Verification items for the finished model (mm, model axes). Face numbers are marked on the shaded views. Coordinates: 2 decimals unless noted, no trailing zeros. Order: outer loops, then holes, each group sorted by start corner. A loop starts at its lowest first (then second) coordinate and runs counter-clockwise, first axis right, second up.
Q1. Depth check by flat-ended pin: P1, Ø6, axis at y = -25.5, z = 115.5, coming from the -X side; P2, Ø12, axis at x = 0, y = 10.5, coming from the +Z side; P3, Ø6, axis at y = -17.5, z = 46, coming from the -X side. Enter the tip coordinate at first touch or a pass-through.
Q2. Thickness scan on line 1 (Y direction, x = 0, z = 47); line 2 (X direction, y = 2.5, z = 117.5); line 3 (X direction, y = 16, z = 34.5). Record the ranges inside material, lowest first.
Q3. Draft check along Y on the marked faces 1, 2 and 3. Enter one of: pulls with the +Y half, pulls with the -Y half, needs draft (parallel to the pull), parting line crosses it, or undercut.
Q4. Cross-section at A-A, the plane z = 116.5. Record the boundary of the cut face in (x, y).
from build123d import *

# Parameters (mm, degrees)
F2_R     = 25
F2_R_2   = 19.999999553
F5_DEPTH = 5
F6_R     = 4.999


# Not quite as in the source:
# - a fillet or chamfer is up to 0.001 mm smaller than in the source, because OpenCascade refuses the exact size


with BuildPart() as f4:
    # F4: sweep along a path in F3
    with BuildLine(Plane.XZ) as f4_path:
        Line((0, 150.3136307001), (0, 0))
    # F2 (on offset) → F4 (sweep)
    with BuildSketch(Plane.XY.offset(150)):
        with Locations((0, 3.1161449583)):
            Circle(F2_R)
        with Locations((0, 3.1161449583)):
            Circle(F2_R_2, mode=Mode.SUBTRACT)
    sweep(path=f4_path.line)

    # F0 (on Top) → F5 (join)
    with BuildSketch(Plane.XY):
        with BuildLine():
            add(Edge.make_bspline(
                [(150, 0), (150, 86.6025403784), (-75, 43.3012701892), (-300, 0), (-75, -43.3012701892), (150, -86.6025403784), (150, 0)],
                knots=[0, 0, 0, 2.0943951024, 2.0943951024, 4.1887902048, 4.1887902048, 6.2831853072, 6.2831853072, 6.2831853072], degree=2, weights=[1, 0.5, 1, 0.5, 1, 0.5, 1]))
        make_face()
    extrude(amount=F5_DEPTH)

    # F6 (radius 5 in the source; OpenCascade refuses exactly that, so slightly less here)
    f6_edges = [f4.edges().sort_by_distance(p)[0] for p in [
        (-150, 0.000863, 5),
        (-25, 3.116145, 5),
    ]]
    fillet(f6_edges, radius=F6_R)


solid = f4.part
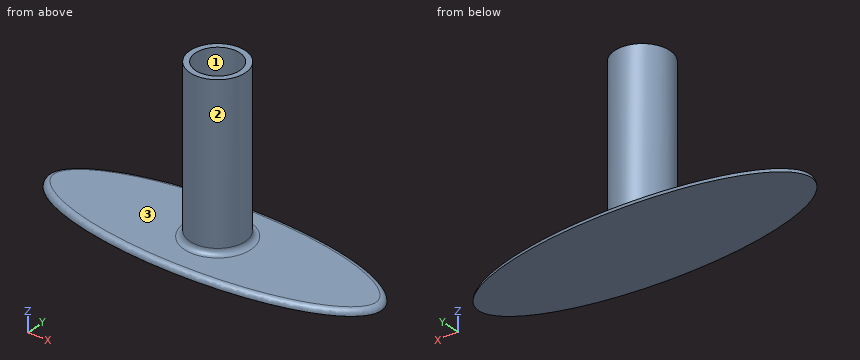
Check values:
1. P1: passes through
1. P2: stops at z = 5
1. P3: stops at x = -17.74
2. line 1: y = -21.88 to -16.88, 23.12 to 28.12
2. line 2: x = -24.99 to -19.99, 19.99 to 24.99
2. line 3: x = -21.42 to -15.3, 15.3 to 21.42
3. face 1: undercut
3. face 2: parting line crosses it
3. face 3: needs draft
4. outline: circle Ø50 at (0, 3.12); hole circle Ø40 at (0, 3.12)
